Geometry check sheet. Reference: the model listing, model coordinates, mm. A direction names the side the tool comes from. Round coordinates to 2 decimals unless told otherwise and drop trailing zeros. Order: outer loops, then holes, each group sorted by start corner. A loop starts at its lowest first (then second) coordinate and runs counter-clockwise, first axis right, second up. Notation, with made-up numbers: (39.5, 79.25) - (43.5, 79.25) arc R23 cw to (43.5, 95.25) - close; hole circle Ø9 at (33.25, 46). An arc over 180 degrees is marked (long way). Return JSON: item names as keys, results as strings. Group by question number.
Q1. Sectioned sample at D-D, the plane z = -23.25. Record the cut outline in (x, y), then the cut area to 3 significant figures.
Q2. Gauge pin test, flat end, axial feed: pin 1 Ø3.5 at (x, y) = (10.5, -4) entering from +Z. Record the tip position at first contact, or that the pin passes through.
Q3. Sectioned sample at A-A, the plane z = -16. Record the cut outline in (x, y).
Q4. Material ranges on line 1 along X through (y, z) = (-3, -22); line 2 along Z through (x, y) = (0.5, -5.75); line 3 along X through (y, z) = (-2.75, -14), recorded low to high.
Q5. Tool access check on faces 5 (the cylindrical face through (-21.833, -3.549, -13.591)), 6 (the flat face through (-22, -3, -15.29)), 7 (the cylindrical face through (30.451, -3.549, -13.575)). Record the directions out of +Z, -Z, +X, -X, +Y, -Y that give a thin tool (end or side, any length) a straight path to the whole face; none if there is none.
Q6. Sectioned sample at C-C, the plane x = 14. Record the cut outline in (y, z), then the cut area to 3 significant figures.
Q7. Draft check along X on faces 1 (the cylindrical face through (-22.978, -3.549, -27.689)), 2 (the flat face through (3, -3, -28.29)), 3 (the cylindrical face through (30.15, -3.55, -27.72)), 4 (the flat face through (28.752, -3, -21)). Enter one of: pulls with the +X half, pulls with the -X half, needs draft (parallel to the pull), parting line crosses it, or undercut.
```python
from build123d import *

# Parameters (mm, degrees)
F1_DEPTH = 7
F2_R     = 2
F3_R     = 1
F4_R     = 0.99999


# Not quite as in the source:
# - a fillet or chamfer is up to 0.001 mm smaller than in the source, because OpenCascade refuses the exact size


with BuildPart() as f1:
    # F0 (on Front) → F1 (new body)
    with BuildSketch(Plane.XZ):
        Polygon((-21.5481998797, -13.2900460566), (-23.5481998797, -13.2900460566), (-23.5481998797, -28.2900460566), (30.7518001203, -28.2900460566), (30.7518001203, -13.2900460566), (28.7518001203, -13.2900460566), (28.7518001203, -15.2900460566), (30.2518001203, -15.2900460566), (30.2518001203, -17.0800460566), (28.7518001203, -17.0800460566), (28.7518001203, -26.2900460566), (-21.5481998797, -26.2900460566), (-21.5481998797, -17.0800460566), (-23.0481998797, -17.0800460566), (-23.0481998797, -15.2900460566), (-21.5481998797, -15.2900460566), align=None)
    extrude(amount=F1_DEPTH)

    # F2
    f2_edges = [f1.edges().sort_by_distance(p)[0] for p in [
        (-23.5482, -3.5, -28.290046),
        (30.7518, -3.5, -28.290046),
    ]]
    fillet(f2_edges, radius=F2_R)

    # F3
    f3_edges = [f1.edges().sort_by_distance(p)[0] for p in [
        (-21.5482, -3.5, -26.290046),
        (28.7518, -3.5, -26.290046),
    ]]
    fillet(f3_edges, radius=F3_R)

    # F4 (radius 1 in the source; OpenCascade refuses exactly that, so slightly less here)
    f4_edges = [f1.edges().sort_by_distance(p)[0] for p in [
        (-23.5482, -3.5, -13.290046),
        (30.7518, -3.5, -13.290046),
        (-21.5482, -3.5, -13.290046),
        (28.7518, -3.5, -13.290046),
    ]]
    fillet(f4_edges, radius=F4_R)


solid = f1.part
```
Reply:
{
 "1": {"outline": "(-23.55, -7) - (-21.55, -7) - (-21.55, 0) - (-23.55, 0) - close; (28.75, -7) - (30.75, -7) - (30.75, 0) - (28.75, 0) - close", "area": "28.0 mm^2"},
 "2": {"pin 1": "z = -26.29"},
 "3": {"outline": "(-23.55, -7) - (-23.05, -7) - (-23.05, 0) - (-23.55, 0) - close; (30.25, -7) - (30.75, -7) - (30.75, 0) - (30.25, 0) - close"},
 "4": {"line 1": "-23.55 to -21.55, 28.75 to 30.75", "line 2": "-28.29 to -26.29", "line 3": "-23.51 to -21.59, 28.79 to 30.71"},
 "5": {"face 5": "+Z, +Y, -Y", "face 6": "+Y, -Y", "face 7": "+Z, +X, +Y, -Y"},
 "6": {"outline": "(-7, -28.29) - (0, -28.29) - (0, -26.29) - (-7, -26.29) - close", "area": "14.0 mm^2"},
 "7": {"face 1": "pulls with the -X half", "face 2": "needs draft", "face 3": "pulls with the +X half", "face 4": "undercut"}
}
